from build123d import *

# Parameters (mm, degrees)
CUT_EXTRUDE_START   = -4
SKETCH_2_R          = 0.5
CUT_EXTRUDE_1_DEPTH = 4
DOME_1_FACE_RADIUS  = 0.5
DOME_1_HEIGHT       = 0.3


with BuildPart() as part:
    # 草图1 → 旋转2 (revolve)
    with BuildSketch(Plane.XY):
        Polygon((0, 13.2), (0, 0), (0.7, 0), (0.7, 5), (2, 5), (2, 6.5), (1, 6.5), (1, 7.5), (2, 7.5), (2, 9), (1, 9), (1, 10), (2, 10), (2, 11), (0.5, 11), (0.5, 13.2), align=None)
    revolve(axis=Axis((0, 0, 0), (0, 1, 0)))

    # 草图2 → 切除-拉伸1 (cut)
    with BuildSketch(Plane(origin=(0, 0, 0), x_dir=(-1, 0, 0), z_dir=(0, -1, 0)).offset(CUT_EXTRUDE_START)):
        with Locations(Location((0, 0, 0), (0, 0, 180))):
            Circle(SKETCH_2_R)
    extrude(amount=CUT_EXTRUDE_1_DEPTH, mode=Mode.SUBTRACT)

    # 圆顶1: a dome of height H over a round flat face of radius A is a cap of a sphere of radius (A * A + H * H) / (2 * H)
    dome_1_r = (DOME_1_FACE_RADIUS * DOME_1_FACE_RADIUS + DOME_1_HEIGHT * DOME_1_HEIGHT) / (2 * DOME_1_HEIGHT)
    dome_1_base = Plane((0, 13.2, 0), z_dir=(0, 1, 0))
    with Locations(dome_1_base.offset(DOME_1_HEIGHT - dome_1_r)):
        dome_1_ball = Sphere(dome_1_r, mode=Mode.PRIVATE)
    add(split(dome_1_ball, bisect_by=dome_1_base, keep=Keep.TOP, mode=Mode.PRIVATE))


solid = part.part
The model under review builds one solid part; all positions refer to its coordinate system, in mm. A direction names the side the tool comes from. Round coordinates to 2 decimals unless told otherwise and drop trailing zeros. Write each loop counter-clockwise with the first axis right and the second up, starting at its lowest first coordinate (ties: lowest second). Pieces come first, ordered by that corner, then holes. Notation, with made-up numbers: (79, 64) -> (88, 64) arc R7 cw to (88, 70) -> close; hole circle Ø3 at (4.5, -29.5). An arc over 180 degrees is marked (long way). Answer as a JSON object with one key per item and string values.
1. The part is to be moulded in two halves that separate along Z. For faces 1 (the face through (0, 6, 2)), 2 (the face through (0, 4, 0)), 3 (the face through (-0.5, 11, -0.5)), say which applies: pulls with the +Z half, pulls with the -Z half, needs draft (parallel to the pull), parting line crosses it, or undercut.
Results found:
{"face 1": "parting line crosses it", "face 2": "undercut", "face 3": "needs draft"}
2. Clearance check with flat-ended pins moving along their axes: pin 1 (1.2 mm diameter, centred on x = 1, z = -1, fed in from +Y); pin 2 (1.2 mm diameter, centred on x = -1, z = 1, fed in from -Y). State where each tip first meets the part, or that it passes through.
Results found:
{"pin 1": "stops at y = 11", "pin 2": "stops at y = 5"}
3. We need section D-D on z = 1.7. State the section outline as (x, y) points, and give its area (3 significant figures).
Results found:
{"outline": "(-1.05, 5) -> (1.05, 5) -> (1.05, 6.5) -> (-1.05, 6.5) -> close; (-1.05, 7.5) -> (1.05, 7.5) -> (1.05, 9) -> (-1.05, 9) -> close; (-1.05, 10) -> (1.05, 10) -> (1.05, 11) -> (-1.05, 11) -> close", "area": "8.43 mm^2"}
4. Machinability: for faces 4 (the face through (-0.108, 2.028, -0.488)), 5 (the face through (0, 8, 2)), 6 (the face through (0, 7, 1)), 7 (the face through (-0.108, 12.115, 0.488)), which of the approach directions +Z, -Z, +X, -X, +Y, -Y give a long, thin tool a straight path to every point of the face, cutting with its end or side? Answer none if there is none.
Results found:
{"face 4": "-Y", "face 5": "+Y, -Y", "face 6": "none", "face 7": "+Y"}
5. We need section C-C on x = 1.65. State the section outline as (y, z) points.
Results found:
{"outline": "(5, -1.13) -> (6.5, -1.13) -> (6.5, 1.13) -> (5, 1.13) -> close; (7.5, -1.13) -> (9, -1.13) -> (9, 1.13) -> (7.5, 1.13) -> close; (10, -1.13) -> (11, -1.13) -> (11, 1.13) -> (10, 1.13) -> close"}
6. To check wall thickness, follow line 1 along Y through (x, z) = (-0.55, 1.5); line 2 along Z through (x, y) = (0, 1.1). State the ranges of each line that lie inside material, in increasing order.
Results found:
{"line 1": "y = 5 to 6.5, 7.5 to 9, 10 to 11", "line 2": "z = -0.7 to -0.5, 0.5 to 0.7"}
